Autodesk Inventor part; units mm, degrees
ref_plane "YZ Plane" through (0, 0, 0) normal (1, 0, 0) x (0, 1, 0)
ref_plane "XZ Plane" through (0, 0, 0) normal (0, 1, 0) x (-1, 0, 0)
ref_plane "XY Plane" through (0, 0, 0) normal (0, 0, 1) x (1, 0, 0)
sketch "Sketch1" plane through (0, 0, 0) normal (0, 0, 1) x (1, 0, 0)
  line L0 (2.1651, -3.75) -> (-2.1651, -3.75)
  line L1 (-2.1651, -3.75) -> (-4.3301, 0)
  line L2 (-4.3301, 0) -> (-2.1651, 3.75)
  line L3 (-2.1651, 3.75) -> (2.1651, 3.75)
  line L4 (2.1651, 3.75) -> (4.3301, 0)
  line L5 (4.3301, 0) -> (2.1651, -3.75)
  circle A0 centre (0, 0) radius 2
  line L6 (-6.0622, 0) -> (6.0622, 0) construction
  dimension "d0" = 7.5
  dimension "d1" = 4
extrude "Extrusion1" add sketch "Sketch1" along normal blind 3
properties part number "HexNut M4"
Can you work these out from the model? Positions are in its coordinate system, mm. Round coordinates to 2 decimals unless told otherwise and drop trailing zeros. Loops run counter-clockwise (first coordinate to the right, second up) from the corner with the lowest first, then second, coordinate; pieces in that order, holes last. Notation, with made-up numbers: M 67.25,30.25 L 98.25,30.25 A32 cw 98.25,60.25 Z; hole C 69,73 d11. An arc over 180 degrees is marked long. Answer in a Markdown table with one row per item.
1. If we section it at D-D, the plane x = 2.75: Please give me the cut outline in (y, z).
Established:
| item | result |
|---|---|
| outline | M -2.74,0 L 2.74,0 L 2.74,3 L -2.74,3 Z |
2. Thinking about a two-plate mould opening in Y: for faces 1 (the face through (0, 2, 1)), 2 (the face through (3.232, 1.901, 1.479)), 3 (the face through (2, 1, 3)), 4 (the face through (-3.232, -1.901, 1.479)), which applies, pulls with the +Y half, pulls with the -Y half, needs draft (parallel to the pull), parting line crosses it, or undercut?
Established:
| item | result |
|---|---|
| face 1 | undercut |
| face 2 | pulls with the +Y half |
| face 3 | needs draft |
| face 4 | pulls with the -Y half |
3. If we section it at B-B, the plane y = -1.5: Please give me the cut outline in (x, z).
Established:
| item | result |
|---|---|
| outline | M -3.46,0 L -1.32,0 L -1.32,3 L -3.46,3 Z; M 1.32,0 L 3.46,0 L 3.46,3 L 1.32,3 Z |
4. If we section it at C-C, the plane x = 0: Please give me the cut outline in (y, z), plus the area to 3 significant figures.
Established:
| item | result |
|---|---|
| outline | M -3.75,0 L -2,0 L -2,3 L -3.75,3 Z; M 2,0 L 3.75,0 L 3.75,3 L 2,3 Z |
| area | 10.5 mm² |
5. I'm going to push a flat-ended pin straight in: pin 1 Ø2.5 at (x, y) = (0, 0) entering from +Z. Where does the tip first touch, or does it pass through?
Established:
| item | result |
|---|---|
| pin 1 | through |
6. If we section it at A-A, the plane z = 1.9: Please give me the cut outline in (x, y), plus the area to 3 significant figures.
Established:
| item | result |
|---|---|
| outline | M -4.33,0 L -2.17,-3.75 L 2.17,-3.75 L 4.33,0 L 2.17,3.75 L -2.17,3.75 Z; hole C 0,0 d4 |
| area | 36.1 mm² |
7. Please list where these lines run through material, in increasing order: line 1 (Y direction, x = 0, z = 0.6); line 2 (X direction, y = 1.5, z = 1.6); line 3 (Y direction, x = -0.5, z = 2.65). Write a range as from..to.
Established:
| item | result |
|---|---|
| line 1 | -3.75..-2, 2..3.75 |
| line 2 | -3.46..-1.32, 1.32..3.46 |
| line 3 | -3.75..-1.94, 1.94..3.75 |
